Check sheet for the modelled part. Datum: model origin and axes. Units: mm. A direction names the side the tool comes from. Round coordinates to 2 decimals unless told otherwise and drop trailing zeros. Order: outer loops, then holes, each group sorted by start corner. A loop starts at its lowest first (then second) coordinate and runs counter-clockwise, first axis right, second up. Notation, with made-up numbers: (47.5, 80.5) -> (65.5, 80.5) arc R27 cw to (65.5, 102.5) -> close; hole circle Ø8 at (86.5, 0.25). An arc over 180 degrees is marked (long way). Answer in a Markdown table with one row per item. Add a question column.
1. Sectioned sample at A-A, the plane y = -22. Record the boundary of the cut face in (x, z), then the cut area to 3 significant figures.
2. Material ranges on L1, parallel to X at y = 26.5, z = 0.4; L2, parallel to X at y = 21, z = 1.1; L3, parallel to Y at x = 16, z = 1.85, recorded low to high. Write a range as from..to.
3. Access from +Z, -Z, +X, -X, +Y, -Y to the whole of each face (thin tool, end or side, straight path). Record for faces 4 (the flat face through (33, 4, 2)), 5 (the flat face through (33, 20, 2)), 6 (the flat face through (16, 26, 2)).
4. Draft check along Y on faces 1 (the flat face through (16, -26, 2)), 2 (the flat face through (-34.3, 16, 2)), 3 (the flat face through (33, -12, 2)). Enter one of: +Y half, -Y half, draft (parallel to the pull), parting line (faces both ways), or undercut.
5. Sectioned sample at B-B, the plane x = -0.5. Record the boundary of the cut face in (y, z).
6. Depth check by flat-ended pin: P1, Ø1.6, axis at y = -23.5, z = 1.5, coming from the +X side; P2, Ø1.6, axis at y = 25, z = 1, coming from the -X side; P3, Ø1.6, axis at x = 33.5, z = 1.5, coming from the -Y side. Enter the tip coordinate at first touch or a pass-through.
```python
from build123d import *

# Parameters (mm, degrees)
ESQUISSE1_W                    = 62
ESQUISSE1_H                    = 52
BOSS_EXTRU_1_DEPTH             = 3.3
ESQUISSE2_W                    = 8
ESQUISSE2_H                    = 3.3
BOSS_EXTRU_2_DEPTH             = 3.3
R_P_TITION_LIN_AIRE1_COUNT     = 2
R_P_TITION_LIN_AIRE1_PITCH     = 16
R_P_TITION_LIN_AIRE1_COL_COUNT = 3
R_P_TITION_LIN_AIRE1_COL_PITCH = 16
SYM_TRIE1_COPY_1_SKETCH_W      = 8
SYM_TRIE1_COPY_1_SKETCH_H      = 3.3
SYM_TRIE1_COPY_1_DEPTH         = 3.3
SYM_TRIE1_COPY_2_SKETCH_W      = 8
SYM_TRIE1_COPY_2_SKETCH_H      = 3.3
SYM_TRIE1_COPY_2_DEPTH         = 3.3
SYM_TRIE1_COPY_3_SKETCH_W      = 8
SYM_TRIE1_COPY_3_SKETCH_H      = 3.3
SYM_TRIE1_COPY_3_DEPTH         = 3.3
ESQUISSE3_W                    = 3
ESQUISSE3_H                    = 3.3
BOSS_EXTRU_3_DEPTH             = 3.3
ESQUISSE4_W                    = 3.3
ESQUISSE4_H                    = 8
BOSS_EXTRU_4_DEPTH             = 3.3
R_P_TITION_LIN_AIRE2_COUNT     = 2
R_P_TITION_LIN_AIRE2_PITCH     = 16
R_P_TITION_LIN_AIRE2_COL_COUNT = 2
R_P_TITION_LIN_AIRE2_COL_PITCH = 16
SYM_TRIE3_COPY_1_SKETCH_W      = 3.3
SYM_TRIE3_COPY_1_SKETCH_H      = 8
SYM_TRIE3_COPY_1_DEPTH         = 3.3
SYM_TRIE3_COPY_2_SKETCH_W      = 3.3
SYM_TRIE3_COPY_2_SKETCH_H      = 8
SYM_TRIE3_COPY_2_DEPTH         = 3.3


with BuildPart() as part:
    # Esquisse1 → Boss.-Extru.1 (new body)
    with BuildSketch(Plane.XY):
        Rectangle(ESQUISSE1_W, ESQUISSE1_H)
    extrude(amount=BOSS_EXTRU_1_DEPTH)

    # Esquisse2 → Boss.-Extru.2 (add)
    with BuildSketch(Plane.XY.offset(3.3)):
        with Locations((8, -27.65)):
            Rectangle(ESQUISSE2_W, ESQUISSE2_H)
    boss_extru_2 = extrude(amount=-BOSS_EXTRU_2_DEPTH)

    # Répétition linéaire1: Boss.-Extru.2 ×2
    with Locations(*[(i * R_P_TITION_LIN_AIRE1_PITCH, 0, 0) for i in range(1, R_P_TITION_LIN_AIRE1_COUNT)]):
        add(boss_extru_2)

    # Répétition linéaire1 col: Boss.-Extru.2 ×3
    with Locations(*[(-i * R_P_TITION_LIN_AIRE1_COL_PITCH, 0, 0) for i in range(1, R_P_TITION_LIN_AIRE1_COL_COUNT)]):
        add(boss_extru_2)

    # Symétrie1: Boss.-Extru.2 across plane
    add(boss_extru_2.mirror(Plane.ZX))

    # Symétrie1 copy 1 sketch → Symétrie1 copy 1 (add)
    with BuildSketch(Plane(origin=(16, 0, 3.3), x_dir=(1, 0, 0), z_dir=(0, 0, 1))):
        with Locations((8, 27.65)):
            Rectangle(SYM_TRIE1_COPY_1_SKETCH_W, SYM_TRIE1_COPY_1_SKETCH_H)
    extrude(amount=-SYM_TRIE1_COPY_1_DEPTH)

    # Symétrie1 copy 2 sketch → Symétrie1 copy 2 (add)
    with BuildSketch(Plane(origin=(-16, 0, 3.3), x_dir=(1, 0, 0), z_dir=(0, 0, 1))):
        with Locations((8, 27.65)):
            Rectangle(SYM_TRIE1_COPY_2_SKETCH_W, SYM_TRIE1_COPY_2_SKETCH_H)
    extrude(amount=-SYM_TRIE1_COPY_2_DEPTH)

    # Symétrie1 copy 3 sketch → Symétrie1 copy 3 (add)
    with BuildSketch(Plane(origin=(-32, 0, 3.3), x_dir=(1, 0, 0), z_dir=(0, 0, 1))):
        with Locations((8, 27.65)):
            Rectangle(SYM_TRIE1_COPY_3_SKETCH_W, SYM_TRIE1_COPY_3_SKETCH_H)
    extrude(amount=-SYM_TRIE1_COPY_3_DEPTH)

    # Esquisse3 → Boss.-Extru.3 (add)
    with BuildSketch(Plane.XY.offset(3.3)):
        with Locations((-29.5, 27.65)):
            Rectangle(ESQUISSE3_W, ESQUISSE3_H)
        with Locations((29.5, 27.65)):
            Rectangle(ESQUISSE3_W, ESQUISSE3_H)
    boss_extru_3 = extrude(amount=-BOSS_EXTRU_3_DEPTH)

    # Symétrie2: Boss.-Extru.3 across plane
    add(boss_extru_3.mirror(Plane.ZX))

    # Esquisse4 → Boss.-Extru.4 (add)
    with BuildSketch(Plane.XY.offset(3.3)):
        with Locations((-32.65, 0)):
            Rectangle(ESQUISSE4_W, ESQUISSE4_H)
    boss_extru_4 = extrude(amount=-BOSS_EXTRU_4_DEPTH)

    # Répétition linéaire2: Boss.-Extru.4 ×2
    with Locations(*[(0, i * R_P_TITION_LIN_AIRE2_PITCH, 0) for i in range(1, R_P_TITION_LIN_AIRE2_COUNT)]):
        add(boss_extru_4)

    # Répétition linéaire2 col: Boss.-Extru.4 ×2
    with Locations(*[(0, -i * R_P_TITION_LIN_AIRE2_COL_PITCH, 0) for i in range(1, R_P_TITION_LIN_AIRE2_COL_COUNT)]):
        add(boss_extru_4)

    # Symétrie3: Boss.-Extru.4 across plane
    add(boss_extru_4.mirror(Plane(origin=(0, 0, 0), x_dir=(0, 0, 1), z_dir=(1, 0, 0))))

    # Symétrie3 copy 1 sketch → Symétrie3 copy 1 (add)
    with BuildSketch(Plane(origin=(0, 16, 3.3), x_dir=(-1, 0, 0), z_dir=(0, 0, 1))):
        with Locations((-32.65, 0)):
            Rectangle(SYM_TRIE3_COPY_1_SKETCH_W, SYM_TRIE3_COPY_1_SKETCH_H)
    extrude(amount=-SYM_TRIE3_COPY_1_DEPTH)

    # Symétrie3 copy 2 sketch → Symétrie3 copy 2 (add)
    with BuildSketch(Plane(origin=(0, -16, 3.3), x_dir=(-1, 0, 0), z_dir=(0, 0, 1))):
        with Locations((-32.65, 0)):
            Rectangle(SYM_TRIE3_COPY_2_SKETCH_W, SYM_TRIE3_COPY_2_SKETCH_H)
    extrude(amount=-SYM_TRIE3_COPY_2_DEPTH)


solid = part.part
```
Answer key:
| question | item | result |
|---|---|---|
| 1 | outline | (-31, 0) -> (31, 0) -> (31, 3.3) -> (-31, 3.3) -> close |
| 1 | area | 205 mm² |
| 2 | L1 | x = -31..-20, -12..-4, 4..12, 20..31 |
| 2 | L2 | x = -31..31 |
| 2 | L3 | y = -26..26 |
| 3 | face 4 | +Z, -Z, +X |
| 3 | face 5 | +Z, -Z, +X, +Y |
| 3 | face 6 | +Z, -Z, +Y |
| 4 | face 1 | -Y half |
| 4 | face 2 | draft |
| 4 | face 3 | undercut |
| 5 | outline | (-26, 0) -> (26, 0) -> (26, 3.3) -> (-26, 3.3) -> close |
| 6 | P1 | stops at x = 31 |
| 6 | P2 | stops at x = -31 |
| 6 | P3 | stops at y = -20 |
